For this review, take the finished solid that the model builds, in its own axes (mm). Face numbers are marked on the shaded views. A direction names the side the tool comes from. Give positions to 0.01 mm unless a question says otherwise; leave off trailing zeros. Order: outer loops, then holes, each group sorted by start corner. A loop starts at its lowest first (then second) coordinate and runs counter-clockwise, first axis right, second up.
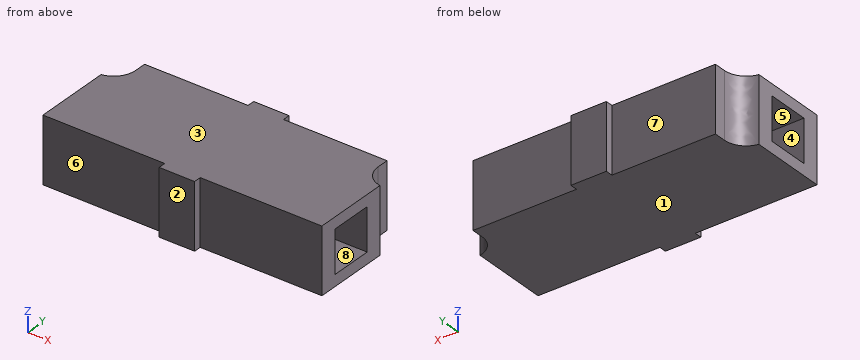
Autodesk Inventor part; units mm, degrees
ref_plane "YZ Plane" through (0, 0, 0) normal (1, 0, 0) x (0, 1, 0)
ref_plane "XZ Plane" through (0, 0, 0) normal (0, 1, 0) x (-1, 0, 0)
ref_plane "XY Plane" through (0, 0, 0) normal (0, 0, 1) x (1, 0, 0)
sketch "Sketch1" plane through (0, 0, 0) normal (0, 0, 1) x (1, 0, 0)
  point P0 (0, 0)
sketch "0" plane through (0, 0, 0) normal (0, 0, 1) x (1, 0, 0)
  spline S0 degree 3 poles (174.458, 140.1191) (175.5599, 140.3052) (176.3666, 141.2594) (176.3666, 142.3769) knots 0 0 0 0 1 1 1 1
  line L0 (174.458, 140.1191) -> (175.5599, 140.3052) construction
  line L1 (175.5599, 140.3052) -> (176.3666, 141.2594) construction
  line L2 (176.3666, 141.2594) -> (176.3666, 142.3769) construction
  spline S1 degree 3 poles (201.7605, 142.3769) (201.7605, 141.2594) (202.5671, 140.3052) (203.6686, 140.1191) knots 0 0 0 0 1 1 1 1
  line L3 (201.7605, 142.3769) -> (201.7605, 141.2594) construction
  line L4 (201.7605, 141.2594) -> (202.5671, 140.3052) construction
  line L5 (202.5671, 140.3052) -> (203.6686, 140.1191) construction
  line L6 (187.2059, 144.3939) -> (189.0634, 144.3939)
  line L7 (187.2059, 144.3939) -> (187.2059, 142.2564)
  line L8 (190.9207, 144.3939) -> (190.9207, 142.9173)
  line L9 (203.6686, 132.066) -> (203.6686, 140.1191)
  line L10 (201.7605, 143.6175) -> (201.7605, 142.3769)
  line L11 (174.458, 132.066) -> (187.2059, 132.066)
  line L12 (176.3666, 143.6175) -> (187.2059, 143.6175)
  line L13 (174.458, 132.066) -> (174.458, 140.1191)
  line L14 (176.3666, 143.6175) -> (176.3666, 142.3769)
  line L15 (203.6686, 132.066) -> (190.9207, 132.066)
  line L16 (201.7605, 143.6175) -> (190.9207, 143.6175)
  line L17 (190.9207, 130.2365) -> (190.9207, 145.2514)
  line L18 (189.0634, 131.2896) -> (189.0634, 144.3939)
  line L19 (189.0634, 131.2896) -> (189.0634, 144.3939)
  line L20 (189.0634, 131.2896) -> (189.0634, 144.3939)
  line L21 (193.4909, 136.8872) -> (192.7376, 136.8872)
  line L22 (192.4867, 136.8872) -> (192.2352, 136.8872)
  line L23 (191.984, 136.8872) -> (190.4774, 136.8872)
  line L24 (190.226, 136.8872) -> (189.9748, 136.8872)
  line L25 (189.7238, 136.8872) -> (188.2172, 136.8872)
  line L26 (187.966, 136.8872) -> (187.7145, 136.8872)
  line L27 (187.4633, 136.8872) -> (185.9567, 136.8872)
  line L28 (185.7055, 136.8872) -> (185.4546, 136.8872)
  line L29 (185.2031, 136.8872) -> (184.4498, 136.8872)
  line L30 (190.9207, 131.2896) -> (189.0634, 131.2896)
  line L31 (187.2059, 131.2896) -> (187.2059, 133.4271)
  line L32 (187.2059, 131.2896) -> (189.0634, 131.2896)
  line L33 (190.9207, 131.2896) -> (190.9207, 132.7662)
  line L34 (190.9207, 144.3939) -> (189.0634, 144.3939)
extrude "Extrusion1" add sketch "0" along normal blind 6.858
sketch "Sketch3" plane through (174.458, 132.066, 0) normal (-1, 0, 0) x (0, 0, 1)
  circle A0 centre (3.429, 4.0386) radius 0.625
  point P0 (0, -132.066)
  dimension "d2" = 1.25
extrude "Extrusion2" cut sketch "Sketch3" against normal through all
sketch "Sketch4" plane through (174.458, 132.066, 0) normal (-1, 0, 0) x (0, 0, 1)
  line L0 (1.194, 6.2736) -> (5.664, 6.2736)
  line L1 (5.664, 6.2736) -> (5.664, 1.8036)
  line L2 (5.664, 1.8036) -> (1.194, 1.8036)
  line L3 (1.194, 1.8036) -> (1.194, 6.2736)
  circle A0 centre (3.429, 4.0386) radius 0.625
  line L4 (1.194, 6.2736) -> (5.664, 1.8036) construction
  line L5 (5.664, 6.2736) -> (1.194, 1.8036) construction
  point P0 (0, -132.066)
  dimension "d5" = 4.47
  dimension "d6" = 4.47
extrude "Extrusion3" cut sketch "Sketch4" against normal blind 10
sketch "Sketch5" plane through (203.6686, 132.066, 0) normal (1, 0, 0) x (0, 0, -1)
  line L0 (-5.664, 1.8036) -> (-1.194, 1.8036)
  line L1 (-5.664, 6.2736) -> (-1.194, 6.2736)
  line L2 (-1.194, 6.2736) -> (-1.194, 1.8036)
  line L3 (-1.194, 1.8036) -> (-5.664, 1.8036)
  line L4 (-5.664, 1.8036) -> (-5.664, 6.2736)
  circle A0 centre (-3.429, 4.0386) radius 0.625
  line L5 (-5.664, 6.2736) -> (-1.194, 1.8036) construction
  line L6 (-1.194, 6.2736) -> (-5.664, 1.8036) construction
  point P0 (0, -132.066)
extrude "Extrusion4" cut sketch "Sketch5" against normal blind 10
properties part number "lc_lc_coupler_molex_1061251100_sd_scaled_3d" material "Acetal Resin, Black"
1) Clearance check with flat-ended pins moving along their axes: pin 1 (0.6 mm diameter, centred on y = 143, z = 4, fed in from +X); pin 2 (0.6 mm diameter, centred on y = 131.5, z = 2, fed in from +X); pin 3 (2 mm diameter, centred on y = 136.1, z = 3.43, fed in from -X). State where each tip first meets the part, or that it passes through.
Answer sheet:
pin 1: stops at x = 201.76
pin 2: stops at x = 190.92
pin 3: stops at x = 184.46
2) To check wall thickness, follow line 1 (Y direction, x = 179.25, z = 4.75); line 2 (Z direction, x = 198.5, y = 134); line 3 (X direction, y = 134.5, z = 5.5). State the ranges of each line that lie inside material, in increasing order.
Answer sheet:
line 1: y = 132.07 to 133.87, 138.34 to 143.62
line 2: z = 0 to 1.19, 5.66 to 6.86
line 3: x = 184.46 to 193.67
3) We need section A-A on x = 198.25. Give the boundary of the cut face in (y, z).
Answer sheet:
outline: (132.07, 0) - (143.62, 0) - (143.62, 6.86) - (132.07, 6.86) - close; hole (133.87, 1.19) - (138.34, 1.19) - (138.34, 5.66) - (133.87, 5.66) - close
4) Tool access review of the marked faces 5, 6, 7 and 8: name each direction out of +Z, -Z, +X, -X, +Y, -Y from which nothing blocks a thin tool from reaching the whole face with its end or side.
Answer sheet:
face 5: -X
face 6: +Z, -Z, -X, -Y
face 7: +Z, -Z, -X, +Y
face 8: +X
5) Draft analysis for pull direction Z (two halves, no side actions). For the marked faces 1, 2, 3 and 4, state which applies: +Z half, -Z half, draft (parallel to the pull), parting line (faces both ways), or undercut.
Answer sheet:
face 1: -Z half
face 2: draft
face 3: +Z half
face 4: undercut
